```python
from build123d import *

# Parameters (mm, degrees)
SKETCH1_W           = 83
SKETCH1_H           = 70
BOSS_EXTRUDE1_DEPTH = 150
SKETCH2_W           = 73
SKETCH2_H           = 290
CUT_EXTRUDE1_DEPTH  = 60
SKETCH3_W           = 290
SKETCH3_H           = 30
CUT_EXTRUDE2_DEPTH  = 109
SKETCH4_W           = 50
SKETCH4_H           = 10
CUT_EXTRUDE3_DEPTH  = 343
SKETCH5_W           = 40
SKETCH5_H           = 15
CUT_EXTRUDE4_DEPTH  = 343


with BuildPart() as part:
    # Sketch1 → Boss-Extrude1 (new, symmetric)
    with BuildSketch(Plane.XY):
        Rectangle(SKETCH1_W, SKETCH1_H)
    extrude(amount=BOSS_EXTRUDE1_DEPTH, both=True)

    # Sketch2 → Cut-Extrude1 (cut)
    with BuildSketch(Plane(origin=(0, 35, 0), x_dir=(1, 0, 0), z_dir=(0, 1, 0))):
        Rectangle(SKETCH2_W, SKETCH2_H)
    extrude(amount=-CUT_EXTRUDE1_DEPTH, mode=Mode.SUBTRACT)

    # Sketch3 → Cut-Extrude2 (cut)
    with BuildSketch(Plane.ZY.offset(41.5)):
        with Locations((0, 20)):
            Rectangle(SKETCH3_W, SKETCH3_H)
    extrude(amount=-CUT_EXTRUDE2_DEPTH, mode=Mode.SUBTRACT)

    # Sketch4 → Cut-Extrude3 (cut)
    with BuildSketch(Plane.XY.offset(150)):
        with Locations((0, 20)):
            Rectangle(SKETCH4_W, SKETCH4_H)
    extrude(amount=-CUT_EXTRUDE3_DEPTH, mode=Mode.SUBTRACT)

    # Sketch5 → Cut-Extrude4 (cut)
    with BuildSketch(Plane(origin=(0, -25, 0), x_dir=(1, 0, 0), z_dir=(0, 1, 0))):
        with Locations((0, 107.5)):
            Rectangle(SKETCH5_W, SKETCH5_H)
    extrude(amount=-CUT_EXTRUDE4_DEPTH, mode=Mode.SUBTRACT)


solid = part.part
```
The model under review builds one solid part; all positions refer to its coordinate system, in mm. A direction names the side the tool comes from. Give positions to 0.01 mm unless a question says otherwise; leave off trailing zeros. Write each loop counter-clockwise with the first axis right and the second up, starting at its lowest first coordinate (ties: lowest second). Pieces come first, ordered by that corner, then holes. Notation, with made-up numbers: (32, 89) - (45, 89) arc R21 cw to (45, 96) - close; hole circle Ø11 at (66.5, 55.25). An arc over 180 degrees is marked (long way). Answer in a Markdown table with one row per item. Add a question column.
1. Tool access review of faces 5 (the flat face through (-1, 0, -150)), 6 (the flat face through (-1, 5, -145)), 7 (the flat face through (0, -30, -115)), 8 (the flat face through (41.5, -16, 2)), 9 (the flat face through (0, 25, -147)): name each direction out of +Z, -Z, +X, -X, +Y, -Y from which nothing blocks a thin tool from reaching the whole face with its end or side.
2. We need section B-B on y = -19. Write out the cut boundary in (x, z), then the cut area to 3 significant figures.
3. Draft analysis for pull direction Z (two halves, no side actions). For faces 1 (the flat face through (-1, 0, 150)), 2 (the flat face through (-1, 35, 148)), 3 (the flat face through (-39, 5, -2)), 4 (the flat face through (-20, -30, -107)), state which applies: +Z half, -Z half, draft (parallel to the pull), parting line (faces both ways), or undercut.
4. Wall thickness on line 1 along Z through (x, y) = (9, 27.5); line 2 along X through (y, z) = (-10, -110); line 3 along Y through (x, z) = (11, -78): over which ranges is each line inside the solid? List them lowest first. Write a range as [from, to].
5. We need section A-A on x = -1. Write out the cut boundary in (y, z), then the cut area to 3 significant figures.
6. We need section D-D on y = 22. Write out the cut boundary in (x, z).
7. We need section C-C on z = -65. Write out the cut boundary in (x, y).
8. Insertion check: P1, Ø8, axis at x = 19.5, z = 92, coming from the +Y side; P2, Ø4, axis at x = -38.5, z = -27, coming from the +Y side; P3, Ø6, axis at y = 5.5, z = 107.5, coming from the +X side. Each pin has a flat end and moves straight along its axis. Give the tip position at first contact, or say it passes through.
Ans:
| question | item | result |
|---|---|---|
| 1 | face 5 | -Z, +X, -X, +Y, -Y |
| 1 | face 6 | +Y |
| 1 | face 7 | +Y, -Y |
| 1 | face 8 | +Z, -Z, +X, +Y, -Y |
| 1 | face 9 | +Z, -Z |
| 2 | outline | (-41.5, -150) - (41.5, -150) - (41.5, 150) - (-41.5, 150) - close; hole (-36.5, -145) - (36.5, -145) - (36.5, 145) - (-36.5, 145) - close |
| 2 | area | 3,730 mm^2 |
| 3 | face 1 | +Z half |
| 3 | face 2 | draft |
| 3 | face 3 | undercut |
| 3 | face 4 | undercut |
| 4 | line 1 | z = [-150, -145], [145, 150] |
| 4 | line 2 | x = [-41.5, -36.5], [36.5, 41.5] |
| 4 | line 3 | y = [-35, -25] |
| 5 | outline | (-35, -150) - (15, -150) - (15, -145) - (-25, -145) - (-25, -115) - (-35, -115) - close; (-35, -100) - (-25, -100) - (-25, 145) - (15, 145) - (15, 150) - (-35, 150) - close; (25, -150) - (35, -150) - (35, -145) - (25, -145) - close; (25, 145) - (35, 145) - (35, 150) - (25, 150) - close |
| 5 | area | 3,350 mm^2 |
| 6 | outline | (-41.5, -150) - (-25, -150) - (-25, -145) - (-41.5, -145) - close; (-41.5, 145) - (-25, 145) - (-25, 150) - (-41.5, 150) - close; (25, -150) - (41.5, -150) - (41.5, -145) - (25, -145) - close; (25, 145) - (41.5, 145) - (41.5, 150) - (25, 150) - close |
| 7 | outline | (-41.5, -35) - (41.5, -35) - (41.5, 5) - (36.5, 5) - (36.5, -25) - (-36.5, -25) - (-36.5, 5) - (-41.5, 5) - close |
| 8 | P1 | stops at y = -25 |
| 8 | P2 | stops at y = 5 |
| 8 | P3 | stops at x = 41.5 |
